Input: part model. Units: mm. Frame: model coordinates. A direction names the side the tool comes from. Coordinates: 2 decimals unless noted, no trailing zeros. Write each loop counter-clockwise with the first axis right and the second up, starting at its lowest first coordinate (ties: lowest second). Pieces come first, ordered by that corner, then holes. Notation, with made-up numbers: M -16.75,51.25 L 41.25,51.25 A24 cw 41.25,87.25 Z; hole C 85.25,41.5 d4. An arc over 180 degrees is marked long. Use one line per item in the form item = value.
Autodesk Inventor part; units mm, degrees
ref_plane "YZ Plane" through (0, 0, 0) normal (1, 0, 0) x (0, 1, 0)
ref_plane "XZ Plane" through (0, 0, 0) normal (0, 1, 0) x (-1, 0, 0)
ref_plane "XY Plane" through (0, 0, 0) normal (0, 0, 1) x (1, 0, 0)
sketch "Sketch1" plane through (0, 0, 0) normal (0, 1, 0) x (-1, 0, 0)
  line L0 (71.1097, -38.0648) -> (71.1097, -13.0648)
  line L1 (71.1097, -13.0648) -> (74.1097, -13.0648)
  line L2 (74.1097, -13.0648) -> (74.1097, 11.9352)
  line L3 (74.1097, 11.9352) -> (71.1097, 11.9352)
  line L4 (71.1097, 11.9352) -> (71.1097, 36.9352)
  line L5 (-72.8903, -38.0648) -> (-72.8903, -13.0648)
  line L6 (-72.8903, 36.9352) -> (-72.8903, 11.9352)
  line L7 (-72.8903, -13.0648) -> (-75.8903, -13.0648)
  line L8 (-75.8903, -13.0648) -> (-75.8903, 11.9352)
  line L9 (-75.8903, 11.9352) -> (-72.8903, 11.9352)
  line L10 (71.1097, -38.0648) -> (-72.8903, -38.0648)
  line L11 (71.1097, 36.9352) -> (-72.8903, 36.9352)
  point P0 (0, 0)
extrude "Extrusion1" add sketch "Sketch1" along normal blind 3
sketch "Sketch2" plane through (0, 3, 0) normal (0, 1, 0) x (1, 0, 0)
  line L0 (-74.1097, 13.0648) -> (-74.1097, -11.9352)
  line L1 (75.8903, -11.9352) -> (75.8903, 13.0648)
  line L2 (-71.1097, -36.9352) -> (72.8903, -36.9352)
  line L3 (-24.1097, -36.9352) -> (25.8903, -36.9352)
  line L4 (25.8903, -36.9352) -> (25.8903, -33.9352)
  line L5 (25.8903, -33.9352) -> (-24.1097, -33.9352)
  line L6 (-24.1097, -33.9352) -> (-24.1097, -36.9352)
  line L7 (72.8903, 38.0648) -> (-71.1097, 38.0648)
  point P0 (0, 0)
  dimension "d13" = 50
  dimension "d14" = 3
extrude "Extrusion2" cut sketch "Sketch2" against normal blind 30
sketch "Sketch3" plane through (0, 3, 0) normal (0, 1, 0) x (1, 0, 0)
  line L0 (-71.1097, -36.9352) -> (-24.1097, -36.9352)
  line L1 (-74.1097, 13.0648) -> (-74.1097, -11.9352)
  line L2 (-54.9097, 25.4648) -> (-64.9114, 25.4648)
  line L3 (-64.9114, 25.4648) -> (-64.9114, -24.8352)
  line L4 (-64.9114, -24.8352) -> (-54.9097, -24.8352)
  line L5 (-54.9097, -24.8352) -> (-54.9097, 25.4648)
  line L6 (56.6903, 25.4648) -> (66.6903, 25.4648)
  line L7 (66.6903, 25.4648) -> (66.6903, -24.8352)
  line L8 (66.6903, -24.8352) -> (56.6903, -24.8352)
  line L9 (56.6903, -24.8352) -> (56.6903, 25.4648)
  circle A0 centre (-34.6697, 22.9248) radius 2
  circle A1 centre (-35.9397, -22.2952) radius 2
  circle A2 centre (40.2603, 22.9248) radius 2
  circle A3 centre (46.6103, -22.2952) radius 2
  line L10 (-49.9097, 28.4648) -> (51.6903, 28.4648)
  line L11 (51.6903, 28.4648) -> (51.6903, 33.4648)
  line L12 (51.6903, 33.4648) -> (-49.9097, 33.4648)
  line L13 (-49.9097, 33.4648) -> (-49.9097, 28.4648)
  point P0 (0, 0)
  dimension "d32" = 4
  dimension "d35" = 4
  dimension "d38" = 4
  dimension "d39" = 4
extrude "Extrusion3" cut sketch "Sketch3" against normal blind 10
sketch "Sketch4" plane through (0, 3, 0) normal (0, 1, 0) x (1, 0, 0)
  circle A0 centre (-34.6697, 22.9248) radius 2
  circle A1 centre (-34.6697, 22.9248) radius 2
  circle A2 centre (40.2603, 22.9248) radius 2
  circle A3 centre (40.2603, 22.9248) radius 2
  circle A4 centre (46.6103, -22.2952) radius 2
  circle A5 centre (46.6103, -22.2952) radius 2
  circle A6 centre (-35.9397, -22.2952) radius 2
  circle A7 centre (-35.9397, -22.2952) radius 2
  point P0 (0, 0)
extrude "Extrusion4" add sketch "Sketch4" against normal blind 3
sketch "Sketch5" plane through (-49.9097, 3, -28.4648) normal (1, 0, 0) x (0, 0, -1)
  line L0 (0, 0) -> (5, 0)
  line L1 (0, 0) -> (5, 0)
  line L2 (5, 0) -> (5, -3)
  line L3 (5, -3) -> (0, -3)
  line L4 (0, -3) -> (0, 0)
  point P0 (-28.4648, -3)
extrude "Extrusion5" add sketch "Sketch5" along normal blind 102.075
properties part number "Level2 (Arduino)"
(1) Line query: probe 1 along X at (y, z) = (0.2, 15); probe 2 along X at (y, z) = (2.45, -12); probe 3 along Z at (x, y) = (-58, 0.25). Output: solid intervals per line, ascending.
Computed:
probe_1 = -71.11 to -64.91, -54.91 to 56.69, 66.69 to 72.89
probe_2 = -74.11 to -64.91, -54.91 to 56.69, 66.69 to 75.89
probe_3 = -38.06 to -25.46, 24.84 to 36.94
(2) Pull-direction query (Z, two-part tool) for faces 1 (the flat face through (49, 1, 36.935)), 2 (the flat face through (-64.911, 2, -1)), 3 (the flat face through (-74.11, 1, -1)); classes: pulls with the +Z half, pulls with the -Z half, needs draft (parallel to the pull), parting line crosses it, or undercut.
Computed:
face_1 = pulls with the +Z half
face_2 = undercut
face_3 = needs draft
(3) Section query C-C on x = -16.5. Return the cut outline in (y, z), plus the area to 3 significant figures.
Computed:
outline = M 0,-38.06 L 3,-38.06 L 3,33.94 L 0,33.94 Z
area = 216 mm^2
(4) Section query A-A on z = -23. Return the cut outline in (x, y).
Computed:
outline = M -71.11,0 L -64.91,0 L -64.91,3 L -71.11,3 Z; M -54.91,0 L 56.69,0 L 56.69,3 L -54.91,3 Z; M 66.69,0 L 72.89,0 L 72.89,3 L 66.69,3 Z
(5) Section query B-B on y = 2.15. Return the cut outline in (x, z), plus the area to 3 significant figures.
Computed:
outline = M -74.11,-13.06 L -71.11,-13.06 L -71.11,-38.06 L 72.89,-38.06 L 72.89,-13.06 L 75.89,-13.06 L 75.89,11.94 L 72.89,11.94 L 72.89,36.94 L 25.89,36.94 L 25.89,33.94 L -24.11,33.94 L -24.11,36.94 L -71.11,36.94 L -71.11,11.94 L -74.11,11.94 Z; hole M -64.91,-25.46 L -54.91,-25.46 L -54.91,24.84 L -64.91,24.84 Z; hole M 56.69,-25.46 L 66.69,-25.46 L 66.69,24.84 L 56.69,24.84 Z
area = 9,790 mm^2
(6) First-contact query: pin 1 Ø1 at (y, z) = (1.5, 18) entering from +X; pin 2 Ø1.5 at (y, z) = (2, 24) entering from -X; pin 3 Ø1.5 at (x, y) = (74, 2) entering from -Z; pin 4 Ø4 at (x, z) = (21, 24) entering from -Y. Flat tips, straight axial feed; report the tip coordinate or a pass-through.
Computed:
pin_1 = 72.89
pin_2 = -71.11
pin_3 = -13.06
pin_4 = 0
(7) Set-up query: faces 4 (the flat face through (72.89, 1, -26)), 5 (the flat face through (74, 1, 11.935)), 6 (the flat face through (-24.11, 2, 35)), 7 (the flat face through (-71.11, 1, -26)), 8 (the flat face through (-54.91, 2, 0)). Return all of +Z, -Z, +X, -X, +Y, -Y with unobstructed straight access to the full face (end or side cutting, diameter ignored); none if empty.
Computed:
face_4 = -Z, +X, +Y, -Y
face_5 = +Z, +X, +Y, -Y
face_6 = +Z, +Y, -Y
face_7 = -Z, -X, +Y, -Y
face_8 = +Y, -Y
